The drawing under review shows one solid part. Ordinate dimensions are in mm from its lowest x, y, z. Coordinates: 2 decimals unless noted, no trailing zeros. Write each loop counter-clockwise with the first axis right and the second up, starting at its lowest first coordinate (ties: lowest second). Pieces come first, ordered by that corner, then holes. Notation, with made-up numbers: M 0,40 L 4,40 A26 ccw 4,77 Z; hole C 24.25,-3 d10. An arc over 180 degrees is marked long. Write each question's results on one line, items separated by ' | '. Start each with the question number.
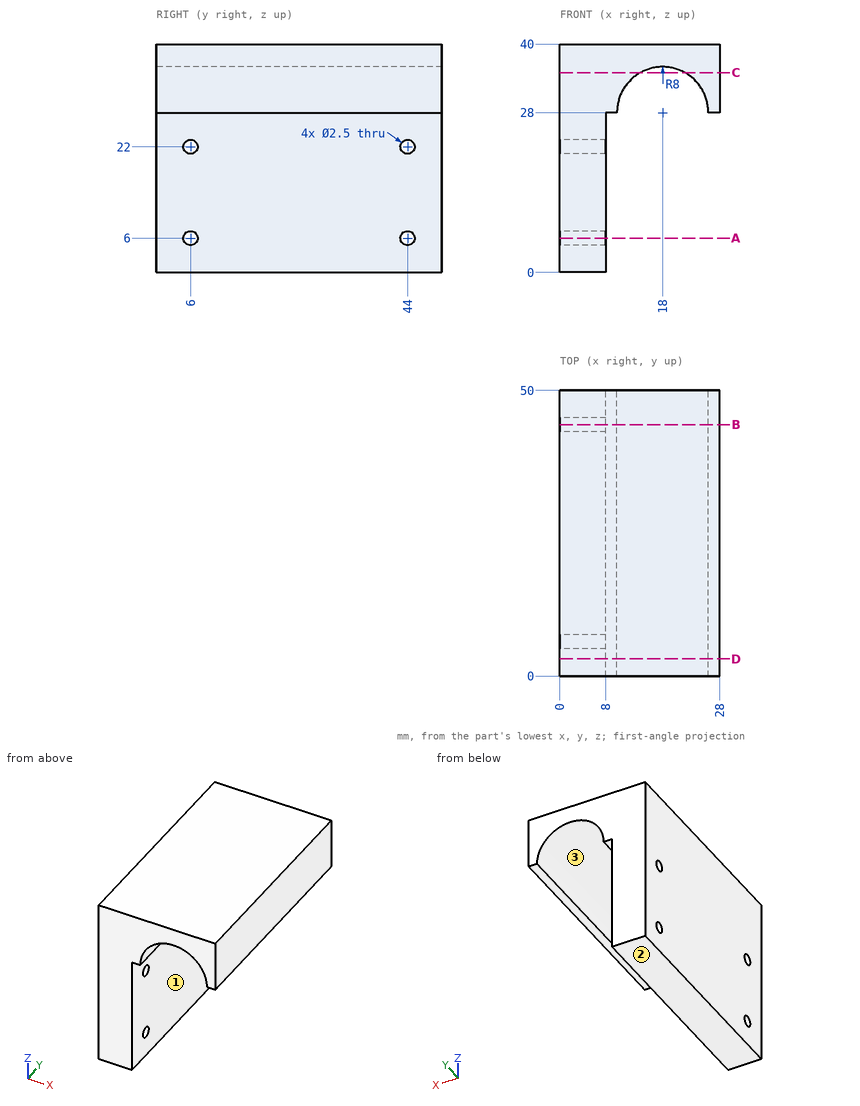
Item 1: Draft analysis for pull direction X (two halves, no side actions). For the marked faces 1, 2 and 3, state which applies: released by +X, released by -X, zero draft, split by the parting line, or undercut.
Item 2: We need section A-A on z = 6. State the section outline as (x, y) points, then the cut area to 3 significant figures.
Item 3: We need section C-C on z = 35. State the section outline as (x, y) points, then the cut area to 3 significant figures.
Item 4: Insertion check: pin 1 Ø1 at (y, z) = (25.5, 28) entering from -X; pin 2 Ø1.6 at (x, y) = (27, 32.5) entering from -Z; pin 3 Ø6 at (y, z) = (25, 21) entering from +X. Each pin has a flat end and moves straight along its axis. Give the tip position at first contact, or say it passes through.
Item 5: We need section D-D on y = 3. State the section outline as (x, z) points.
Item 6: We need section B-B on y = 44. State the section outline as (x, z) points, then the cut area to 3 significant figures.
Item 7: Wall thickness on L1, parallel to Y at x = 3.75, z = 6; L2, parallel to Z at x = 2.5, y = 43.5; L3, parallel to X at y = 3.5, z = 24: over which ranges is each line inside the solid? List them lowest first.
Answer:
1) face 1: released by +X | face 2: zero draft | face 3: undercut
2) outline: M 0,0 L 8,0 L 8,4.75 L 0,4.75 Z; M 0,7.25 L 8,7.25 L 8,42.75 L 0,42.75 Z; M 0,45.25 L 8,45.25 L 8,50 L 0,50 Z | area: 360 mm^2
3) outline: M 0,0 L 14.13,0 L 14.13,50 L 0,50 Z; M 21.87,0 L 28,0 L 28,50 L 21.87,50 Z | area: 1,010 mm^2
4) pin 1: stops at x = 0 | pin 2: stops at z = 28 | pin 3: stops at x = 8
5) outline: M 0,0 L 8,0 L 8,28 L 10,28 A8 cw 26,28 L 28,28 L 28,40 L 0,40 Z
6) outline: M 0,0 L 8,0 L 8,4.75 L 0,4.75 Z; M 0,7.25 L 8,7.25 L 8,20.75 L 0,20.75 Z; M 0,23.25 L 8,23.25 L 8,28 L 10,28 A8 cw 26,28 L 28,28 L 28,40 L 0,40 Z | area: 419 mm^2
7) L1: y = 0 to 4.75, 7.25 to 42.75, 45.25 to 50 | L2: z = 0 to 4.85, 7.15 to 20.85, 23.15 to 40 | L3: x = 0 to 8
